Here's the drawing with two shaded views (mm, measured from the low corner). I have some questions. Round coordinates to 2 decimals unless told otherwise and drop trailing zeros. Order: outer loops, then holes, each group sorted by start corner. A loop starts at its lowest first (then second) coordinate and runs counter-clockwise, first axis right, second up. Notation, with made-up numbers: (-32, -16) -> (18, -16) arc R10 cw to (18, -1) -> close; hole circle Ø2 at (-36, 11.5). An arc over 180 degrees is marked (long way). Answer in a Markdown table with one row per item.
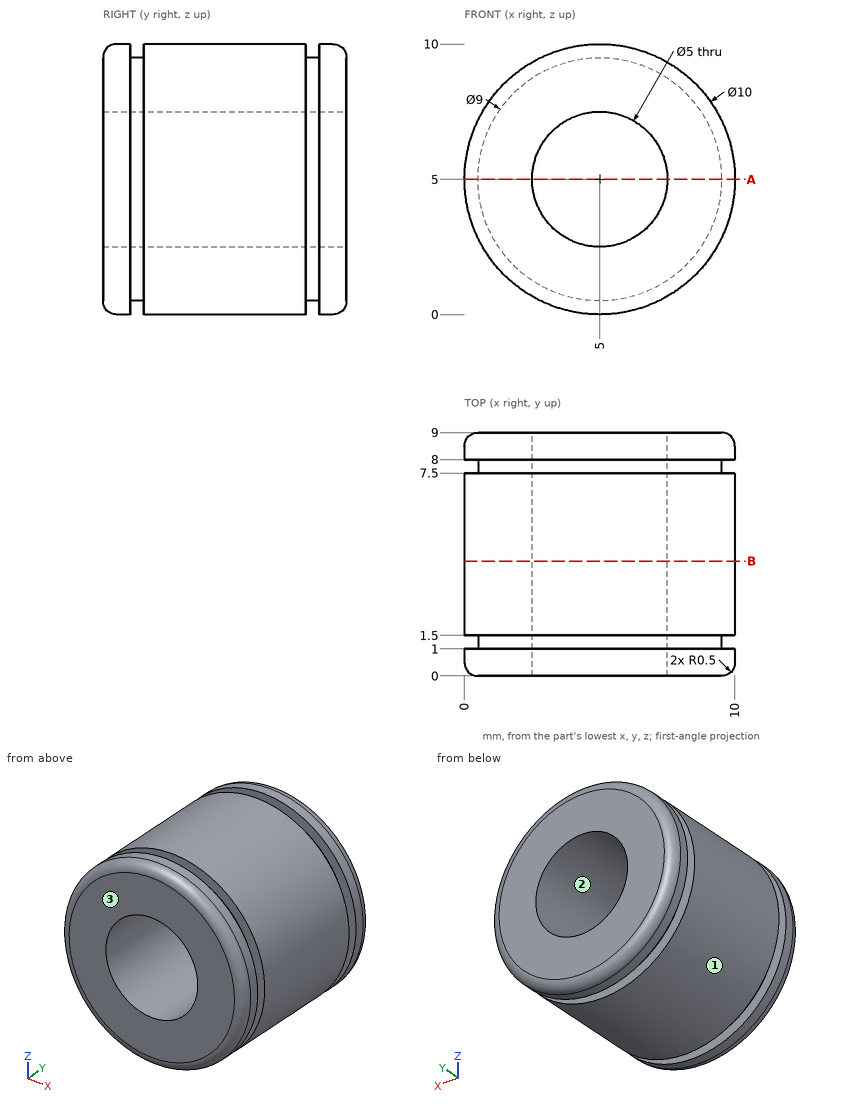
1. For pin 1 Ø1.5 at (y, z) = (6.5, 2.5) entering from +X; pin 2 Ø4 at (y, z) = (1.5, 7.5) entering from +X, each with a flat end and sliding along its axis, tell me the tip position at first contact or that it passes through.
Numbers:
| item | result |
|---|---|
| pin 1 | stops at x = 9.68 |
| pin 2 | stops at x = 9.97 |
2. Please list where these lines run through material, in increasing order: line 1 along X through (y, z) = (2, 5); line 2 along X through (y, z) = (4.5, 6.5).
Numbers:
| item | result |
|---|---|
| line 1 | x = 0 to 2.5, 7.5 to 10 |
| line 2 | x = 0.23 to 3, 7 to 9.77 |
3. Suppose I cut it at A-A on z = 5. Write out the boundary of the cut face in (x, y), then the cut area to 3 significant figures.
Numbers:
| item | result |
|---|---|
| outline | (0, 0.5) arc R0.5 ccw to (0.5, 0) -> (2.5, 0) -> (2.5, 9) -> (0.5, 9) arc R0.5 ccw to (0, 8.5) -> (0, 8) -> (0.5, 8) -> (0.5, 7.5) -> (0, 7.5) -> (0, 1.5) -> (0.5, 1.5) -> (0.5, 1) -> (0, 1) -> close; (7.5, 0) -> (9.5, 0) arc R0.5 ccw to (10, 0.5) -> (10, 1) -> (9.5, 1) -> (9.5, 1.5) -> (10, 1.5) -> (10, 7.5) -> (9.5, 7.5) -> (9.5, 8) -> (10, 8) -> (10, 8.5) arc R0.5 ccw to (9.5, 9) -> (7.5, 9) -> close |
| area | 43.8 mm2 |
4. We'd pull the mould along X, two halves only. Please class the marked faces 1, 2 and 3: released by +X, released by -X, zero draft, split by the parting line, or undercut.
Numbers:
| item | result |
|---|---|
| face 1 | split by the parting line |
| face 2 | undercut |
| face 3 | zero draft |
5. Suppose I cut it at B-B on y = 4.25. Write out the boundary of the cut face in (x, z), then the cut area to 3 significant figures.
Numbers:
| item | result |
|---|---|
| outline | circle Ø10 at (5, 5); hole circle Ø5 at (5, 5) |
| area | 58.9 mm2 |
